```python
from build123d import *

# Parameters (mm, degrees)
F0_W     = 34.6808620631
F0_H     = 50
F1_DEPTH = 10
F2_DEPTH = 50
F3_W     = 125
F3_H     = 10
F4_DEPTH = 25
F5_R     = 10
F6_R     = 5
F7_R     = 5
F8_D     = 3.5
F8_DEPTH = 12
F8_TIP   = 1.0515060833
F9_R     = 4.99999


# Not quite as in the source:
# - a fillet or chamfer is up to 0.001 mm smaller than in the source, because OpenCascade refuses the exact size


with BuildPart() as f1:
    # F0 (on Top) → F1 (new body)
    with BuildSketch(Plane.XY):
        Polygon((-17.3404310315, -25), (-17.3404310315, 25), (-40.2640256677, 25), (-62.5, 25), (-62.5, -25), (-40.2640256677, -25), align=None)
        Polygon((62.5, -25), (62.5, 25), (40.2640256677, 25), (17.3404310315, 25), (17.3404310315, -25), (40.2640256677, -25), align=None)
        Rectangle(F0_W, F0_H)
    extrude(amount=F1_DEPTH)

    # F0 (on Top) → F2 (join)
    with BuildSketch(Plane.XY):
        Rectangle(F0_W, F0_H)
    extrude(amount=F2_DEPTH)

    # F3 (on Front) → F4 (join, symmetric)
    with BuildSketch(Plane.XZ):
        with Locations((0, 49.6251098812)):
            Rectangle(F3_W, F3_H)
    extrude(amount=F4_DEPTH, both=True)

    # F5
    f5_edges = [f1.edges().sort_by_distance(p)[0] for p in [
        (-17.340431, 0, 10),
        (17.340431, 0, 10),
        (17.340431, 0, 44.62511),
        (-17.340431, 0, 44.62511),
    ]]
    fillet(f5_edges, radius=F5_R)

    # F6
    f6_edges = [f1.edges().sort_by_distance(p)[0] for p in [
        (44.920216, -25, 10),
        (44.920216, 25, 10),
        (-44.920216, -25, 10),
        (-44.920216, 25, 10),
    ]]
    fillet(f6_edges, radius=F6_R)

    # F7
    f7_edges = [f1.edges().sort_by_distance(p)[0] for p in [
        (-62.5, 0, 10),
        (-62.5, 0, 44.62511),
        (62.5, 0, 10),
        (62.5, 0, 44.62511),
    ]]
    fillet(f7_edges, radius=F7_R)

    # F8
    with Locations(Plane(origin=(0, 0, 0), x_dir=(1, 0, 0), z_dir=(0, 0, -1))):
        with Locations((-40.2640256677, 0), (40.2640256677, 0)):
            Hole(F8_D / 2, depth=F8_DEPTH)
            with Locations((0, 0, -(F8_DEPTH + F8_TIP / 2))):  # 118° drill point
                Cone(0, F8_D / 2, F8_TIP, mode=Mode.SUBTRACT)

    # F9 (radius 5 in the source; OpenCascade refuses exactly that, so slightly less here)
    f9_edges = [f1.edges().sort_by_distance(p)[0] for p in [
        (0, 25, 54.62511),
        (62.5, 0, 54.62511),
    ]]
    fillet(f9_edges, radius=F9_R)


solid = f1.part
```
Input: part model. Units: mm. Frame: model coordinates. A direction names the side the tool comes from. Round coordinates to 2 decimals unless told otherwise and drop trailing zeros. Loops run counter-clockwise (first coordinate to the right, second up) from the corner with the lowest first, then second, coordinate; pieces in that order, holes last. Notation, with made-up numbers: (77.25, 57) - (117.25, 57) arc R19 ccw to (117.25, 66) - close; hole circle Ø7 at (-30.5, -1.5). An arc over 180 degrees is marked (long way). One line per item, written item: value. Start each with the question number.
(1) Contact query for flat-ended pins moving along their axis: P1, Ø2, axis at y = 9.5, z = 28, coming from the -X side; P2, Ø11.5, axis at y = -0.5, z = 25.5, coming from the +X side; P3, Ø4, axis at y = -17, z = 8, coming from the -X side. Output: stop coordinate, or through.
(2) Section B-B, the plane z = 30. Return loops of the section in (x, y), plus the area to 3 significant figures.
(3) Draft query along Z for faces 1 (the cylindrical face through (61.074, -0.28, 53.122)), 2 (the cylindrical face through (-61.07, 23.5, 2.54)), 3 (the cylindrical face through (-15.84, 23.57, 27.21)), 4 (the flat face through (42, 0, 44.625)). Return one class per face: +Z half, -Z half, draft (parallel to the pull), parting line (faces both ways), or undercut.
(4) Access query for faces 5 (the cylindrical face through (42, 24, 8)), 6 (the flat face through (0, -25, 19)), 7 (the flat face through (17.34, 0, 27)), 8 (the cylindrical face through (-61.074, 0.28, 53.122)), 9 (the flat face through (-43, 0, 44.625)). Directions: +Z, -Z, +X, -X, +Y, -Y. A direction counts if a zero-diameter tool reaches every point of the face in a straight line with its end or side. Return the directions, or none.
(5) Ray query, line 1 (Z direction, x = -37, y = 9); line 2 (X direction, y = -20, z = 22.5); line 3 (Z direction, x = 33, y = -21.5). Return the intervals inside material, ascending. Write a range as [from, to].
(6) Section A-A, the plane y = 0. Count the separate pieces of the cut face and the enclosed holes in it, plus the area to 3 significant figures.
Results below:
1. P1: x = -17.34
1. P2: x = 17.34
1. P3: x = -62.4
2. outline: (-17.34, -20) arc R5 ccw to (-12.34, -25) - (12.34, -25) arc R5 ccw to (17.34, -20) - (17.34, 20) arc R5 ccw to (12.34, 25) - (-12.34, 25) arc R5 ccw to (-17.34, 20) - close
2. area: 1,710 mm^2
3. face 1: +Z half
3. face 2: draft
3. face 3: undercut
3. face 4: undercut
4. face 5: +X, +Y
4. face 6: +Z, -Z, +X, -X, -Y
4. face 7: +X, +Y, -Y
4. face 8: +Z, -X, +Y, -Y
4. face 9: -X, +Y, -Y
5. line 1: [0, 10], [44.63, 54.63]
5. line 2: [-17.34, 17.34]
5. line 3: [0, 9.77], [44.86, 54.39]
6. separate pieces: 3
6. enclosed holes: 0
6. area: 3,680 mm^2
